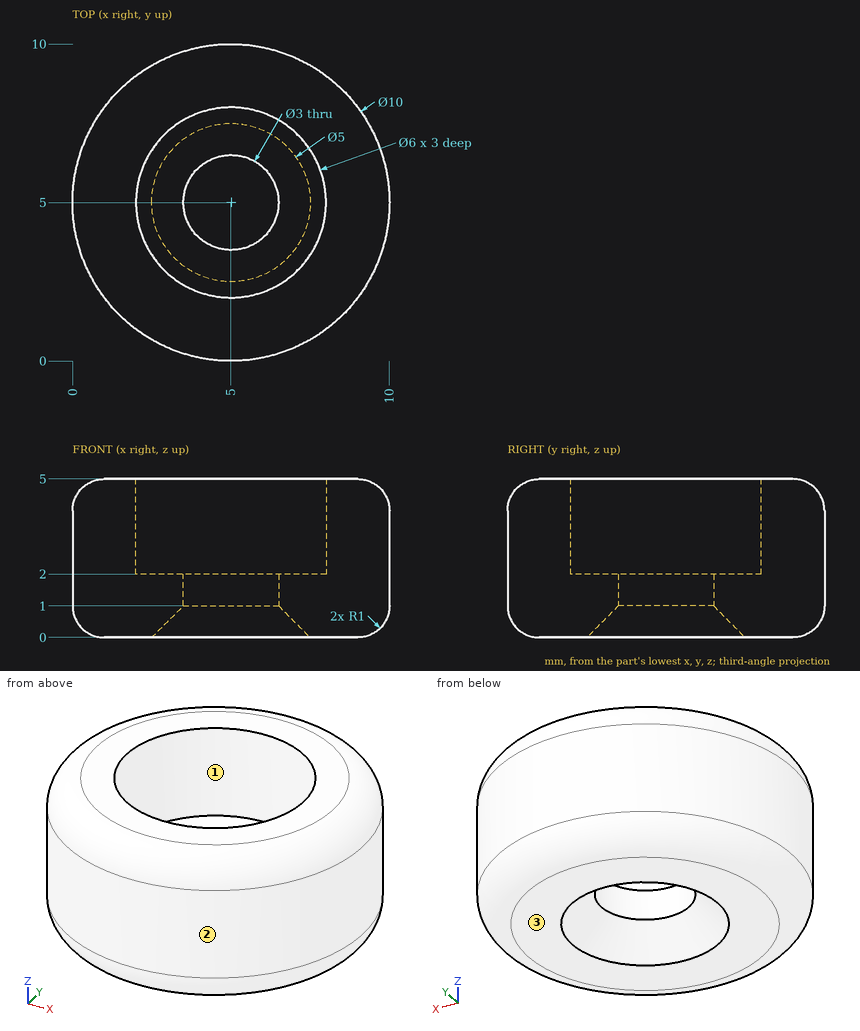
Geometry check sheet. Reference: drawing and pictorial views, mm from the part's lowest x, y, z. Round coordinates to 2 decimals unless told otherwise and drop trailing zeros. Write item = value, one per line. Start each with the question number.
Q1. Release check for a two-part mould opening along Y. For the marked faces 1, 2 and 3 record: pulls with the +Y half, pulls with the -Y half, needs draft (parallel to the pull), parting line crosses it, or undercut.
Q2. Depth check by flat-ended pin: P1, Ø4, axis at x = 8.5, y = 1.5, coming from the -Z side; P2, Ø2, axis at y = 2.5, z = 2.5, coming from the -X side; P3, Ø1, axis at y = 6, z = 3.5, coming from the -X side; P4, Ø2.5, axis at x = 5, y = 5, coming from the +Z side. Enter the tip coordinate at first touch or a pass-through.
Q3. Thickness scan on L1, parallel to Y at x = 5, z = 1.8; L2, parallel to Y at x = 5.25, z = 2.9; L3, parallel to X at y = 7.75, z = 3.25. Record the ranges inside material, lowest first.
Derived:
q1.face_1 = undercut
q1.face_2 = parting line crosses it
q1.face_3 = needs draft
q2.P1 = 0
q2.P2 = 0.23
q2.P3 = 0.03
q2.P4 = through
q3.L1 = 0 to 3.5, 6.5 to 10
q3.L2 = 0.01 to 2.01, 7.99 to 9.99
q3.L3 = 0.82 to 3.8, 6.2 to 9.18
